The listing builds one solid part. Answer for the finished solid, in the listing's coordinates (mm). A direction names the side the tool comes from. Round coordinates to 2 decimals unless told otherwise and drop trailing zeros. Write each loop counter-clockwise with the first axis right and the second up, starting at its lowest first coordinate (ties: lowest second). Pieces come first, ordered by that corner, then holes.
(1) Find the intervals of material crossed by probe 1 along X at (y, z) = (4.5, 12.5); probe 2 along X at (y, z) = (2.25, -0.25); probe 3 along Y at (x, z) = (-19, -1.5) (3 decimals), in increasing order.
(2) The mould has two halves that part along Z. Classify faces 1 (the face through (24.448, 2, -11)), 2 (the face through (-25.143, 1.61, 7.39)), 3 (the face through (-23.303, 4.696, -12.722)): +Z half, -Z half, draft (parallel to the pull), parting line (faces both ways), or undercut.
(3) A cutting plane is placed at C-C, the plane x = 25.4. Give the vertices of the cut face in (y, z) (3 decimals).
(4) A cutting plane is placed at B-B, the plane z = 0. Give the vertices of the cut face in (x, y) (3 decimals).
(5) Each of these flat-tipped pins is pushed along its axis until it touches: pin 1 Ø1.4 at (x, z) = (-22.22, 12.38) entering from +Y; pin 2 Ø3 at (y, z) = (2, -10.5) entering from -X; pin 3 Ø3 at (x, z) = (-18.5, 0) entering from +Y (3 decimals); pin 4 Ø3 at (x, y) = (25.5, 6.5) entering from +Z. Where does it stop, or does it pass through?
(6) A cutting plane is placed at D-D, the plane x = -12. Give the vertices of the cut face in (y, z) (3 decimals).
(7) For faces 4 (the face through (-24.448, 2, -11)), 5 (the face through (25.143, 1.61, -7.39)), 6 (the face through (24.448, 2, 11)), 7 (the face through (-24.448, 2, 11)), determine the directions among +Z, -Z, +X, -X, +Y, -Y from which every point of the face is accessible in a straight line to the end or side of a thin tool.
(8) A cutting plane is placed at A-A, the plane y = 4.75. Give the vertices of the cut face in (x, z) (1 decimal), and give its area (3 significant figures).
from build123d import *

# Parameters (mm, degrees)
BOSS_EXTRUDE1_DEPTH    = 3.175
FILLET1_R              = 3.429
F_10_CLEARANCE_HOLE1_D = 5.1054
SKETCH4_R              = 2.2225
BOSS_EXTRUDE2_DEPTH    = 6.35
F_4_40_TAPPED_HOLE1_D  = 2.2606
CUT_EXTRUDE1_DEPTH     = 4.175
MIRROR2_COPY_1_DEPTH   = 4.175


with BuildPart() as part:
    # Sketch1 → Boss-Extrude1 (new body)
    with BuildSketch(Plane(origin=(0, 0, 0), x_dir=(1, 0, 0), z_dir=(0, 1, 0))):
        with BuildLine():
            Line((-24.4475, 14.605), (24.4475, 14.605))
            Line((24.4475, 14.605), (24.4475, 6.278156079))
            ThreePointArc((24.4475, 6.278156079), (31.75, 0), (24.4475, -6.278156079))
            Line((24.4475, -6.278156079), (24.4475, -14.605))
            Line((24.4475, -14.605), (-24.4475, -14.605))
            Line((-24.4475, -14.605), (-24.4475, -6.278156079))
            ThreePointArc((-24.4475, -6.278156079), (-31.75, 0), (-24.4475, 6.278156079))
            Line((-24.4475, 6.278156079), (-24.4475, 14.605))
        make_face()
    extrude(amount=BOSS_EXTRUDE1_DEPTH)

    # Fillet1
    fillet1_edges = [part.edges().sort_by_distance(p)[0] for p in [
        (-24.4475, 1.5875, 6.278156079),
        (-24.4475, 1.5875, -6.278156079),
        (24.4475, 1.5875, -6.278156079),
        (24.4475, 1.5875, 6.278156079),
    ]]
    fillet(fillet1_edges, radius=FILLET1_R)

    # #10 Clearance Hole1 (through all)
    with Locations(Plane(origin=(0, 3.175, 0), x_dir=(1, 0, 0), z_dir=(0, 1, 0))):
        with Locations((25.4, 0), (-25.4, 0)):
            Hole(F_10_CLEARANCE_HOLE1_D / 2)

    # Sketch4 → Boss-Extrude2 (add)
    with BuildSketch(Plane(origin=(0, 3.175, 0), x_dir=(1, 0, 0), z_dir=(0, 1, 0))):
        with Locations((-22.225, 12.3825)):
            Circle(SKETCH4_R)
        with Locations((22.225, 12.3825)):
            Circle(SKETCH4_R)
        with Locations((22.225, -12.3825)):
            Circle(SKETCH4_R)
        with Locations((-22.225, -12.3825)):
            Circle(SKETCH4_R)
    extrude(amount=BOSS_EXTRUDE2_DEPTH)

    # #4-40 Tapped Hole1 (through all)
    with Locations(Plane(origin=(0, 9.525, 0), x_dir=(1, 0, 0), z_dir=(0, 1, 0))):
        with Locations((22.225, 12.3825), (-22.225, 12.3825), (-22.225, -12.3825), (22.225, -12.3825)):
            Hole(F_4_40_TAPPED_HOLE1_D / 2)

    # Sketch7 → Cut-Extrude1 (cut, through all)
    with BuildSketch(Plane(origin=(0, 3.175, 0), x_dir=(1, 0, 0), z_dir=(0, 1, 0))):
        with BuildLine():
            Line((-24.4475, -14.605), (-22.225, -14.605))
            ThreePointArc((-22.225, -14.605), (-23.796544821, -13.954044821), (-24.4475, -12.3825))
            Line((-24.4475, -12.3825), (-24.4475, -14.605))
        make_face()
    cut_extrude1 = extrude(amount=-CUT_EXTRUDE1_DEPTH, mode=Mode.SUBTRACT)

    # Mirror1: Cut-Extrude1 across plane
    add(cut_extrude1.mirror(Plane.XY), mode=Mode.SUBTRACT)

    # Mirror2: Cut-Extrude1 across plane
    add(cut_extrude1.mirror(Plane(origin=(0, 0, 0), x_dir=(0, 0, 1), z_dir=(1, 0, 0))), mode=Mode.SUBTRACT)

    # Mirror2 copy 1 sketch → Mirror2 copy 1 (cut, through all)
    with BuildSketch(Plane(origin=(0, 3.175, 0), x_dir=(-1, 0, 0), z_dir=(0, 1, 0))):
        with BuildLine():
            Line((-24.4475, -14.605), (-22.225, -14.605))
            ThreePointArc((-22.225, -14.605), (-23.796544821, -13.954044821), (-24.4475, -12.3825))
            Line((-24.4475, -12.3825), (-24.4475, -14.605))
        make_face()
    extrude(amount=-MIRROR2_COPY_1_DEPTH, mode=Mode.SUBTRACT)


solid = part.part
Solutions:
1. probe 1: x = -24.44 to -23.35, -21.1 to -20.01, 20.01 to 21.1, 23.35 to 24.44
1. probe 2: x = -31.75 to -27.94, -22.86 to 22.86, 27.94 to 31.75
1. probe 3: y = 0 to 3.175
2. face 1: draft
2. face 2: +Z half
2. face 3: undercut
3. outline: (0, -7.089) - (3.175, -7.089) - (3.175, -2.553) - (0, -2.553) - close; (0, 2.553) - (3.175, 2.553) - (3.175, 7.089) - (0, 7.089) - close
4. outline: (-31.75, 0) - (-27.953, 0) - (-27.953, 3.175) - (-31.75, 3.175) - close; (-22.847, 0) - (22.847, 0) - (22.847, 3.175) - (-22.847, 3.175) - close; (27.953, 0) - (31.75, 0) - (31.75, 3.175) - (27.953, 3.175) - close
5. pin 1: passes through
5. pin 2: stops at x = -24.48
5. pin 3: stops at y = 3.175
5. pin 4: stops at z = 13.72
6. outline: (0, -14.605) - (3.175, -14.605) - (3.175, 14.605) - (0, 14.605) - close
7. face 4: -Z, -X, +Y, -Y
7. face 5: -Z, +X, +Y, -Y
7. face 6: +Z, +X, +Y, -Y
7. face 7: +Z, -X, +Y, -Y
8. outline: circle Ø4.4 at (-22.2, -12.4); circle Ø4.4 at (-22.2, 12.4); circle Ø4.4 at (22.2, -12.4); circle Ø4.4 at (22.2, 12.4); hole circle Ø2.3 at (-22.2, -12.4); hole circle Ø2.3 at (-22.2, 12.4); hole circle Ø2.3 at (22.2, -12.4); hole circle Ø2.3 at (22.2, 12.4)
8. area: 46.0 mm2
